Geometry check sheet. Reference: the model listing, model coordinates, mm. Face numbers are marked on the shaded views. A direction names the side the tool comes from. Coordinates: 2 decimals unless noted, no trailing zeros. Write each loop counter-clockwise with the first axis right and the second up, starting at its lowest first coordinate (ties: lowest second). Pieces come first, ordered by that corner, then holes. Notation, with made-up numbers: (84, 27) - (124, 27) arc R13 cw to (124, 51) - close; hole circle Ø2 at (-33.5, 89). An arc over 180 degrees is marked (long way). Answer as a JSON object with one key per item and string values. Group by question number.
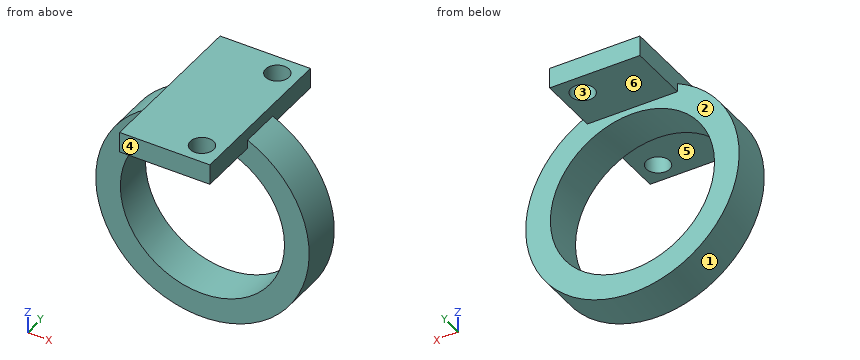
Autodesk Inventor part; units mm, degrees
ref_plane "Work Plane1" through (0, 0, 12) normal (0, 0, 1) x (1, 0, 0)
ref_plane "YZ Plane" through (0, 0, 0) normal (1, 0, 0) x (0, 1, 0)
ref_plane "XZ Plane" through (0, 0, 0) normal (0, 1, 0) x (-1, 0, 0)
sketch "Sketch2" plane through (0, 0, 0) normal (0, 1, 0) x (-1, 0, 0)
  circle A0 centre (0, 0) radius 10
  circle A1 centre (0, 0) radius 13
  dimension "d7" = 20
  dimension "d8" = 26
extrude "Extrusion1" add sketch "Sketch2" along normal blind 5
sketch "Sketch3" plane through (0, 0, 0) normal (0, 0, 1) x (1, 0, 0)
  point P0 (0, 0)
ref_plane "Work Plane1" through (0, 0, 12) normal (0, 0, 1) x (1, 0, 0)
sketch "Sketch4" plane through (0, 0, 12) normal (0, 0, 1) x (1, 0, 0)
  point P0 (0, 0)
sketch "Sketch5" plane through (0, 0, 12) normal (0, 0, 1) x (1, 0, 0)
  line L0 (-13, 0) -> (13, 0)
  line L1 (5.5, 0) -> (-5.5, 0)
  line L2 (-5.5, 0) -> (-5.5, 12.5)
  line L3 (-5.5, 12.5) -> (5.5, 12.5)
  line L4 (5.5, 12.5) -> (5.5, 0)
  line L5 (-5.5, 0) -> (5.5, 0)
  line L6 (5.5, 0) -> (5.5, -7.5)
  line L7 (5.5, -7.5) -> (-5.5, -7.5)
  line L8 (-5.5, -7.5) -> (-5.5, 0)
  line L9 (0, -16.9) -> (0, 20.9)
  dimension "d16" = 11
  dimension "d17" = 7.5
  dimension "d18" = 12.5
  dimension "d19" = 5.5
extrude "Extrusion2" add sketch "Sketch5" along normal mid plane 2.5
sketch "Sketch6" plane through (0, 0, 13.25) normal (0, 0, 1) x (1, 0, 0)
  line L0 (5.5, -7.5) -> (5.5, 12.5)
  line L1 (5.5, 12.5) -> (-5.5, 12.5)
  line L2 (-5.5, -7.5) -> (5.5, -7.5)
  point P0 (0, 0)
  point P1 (3, 10)
  point P2 (3, -5)
  dimension "d20" = 2.5
  dimension "d21" = 2.5
  dimension "d22" = 2.5
  dimension "d30" = 2.5
hole "Hole1" at (3, -5, 13.25) at (3, 10, 13.25) direction (0, 0, -1) diameter 2.85 depth 8 tip angle 118
properties part number "Ring"
(1) Gauge pin test, flat ends, axial feed: pin 1 (1.5 mm diameter, centred on y = 0, z = 7.5, fed in from +X); pin 2 (7.5 mm diameter, centred on x = -2, z = -6.5, fed in from +Y); pin 3 (2 mm diameter, centred on y = 3.5, z = -9, fed in from -X). Record the tip position at first contact, or that the pin passes through.
(2) Draft check along X on the marked faces 1, 2 and 3. Enter one of: +X half, -X half, draft (parallel to the pull), parting line (faces both ways), or undercut.
(3) Section check C-C (z = 0). Record the cut outline in (x, y), and give its area (3 significant figures).
(4) Section check D-D (x = 3). Record the cut outline in (y, z) (3 decimals), and give its area (3 significant figures).
(5) Section check A-A (x = 0). Record the cut outline in (y, z).
(6) Material ranges on L1, parallel to Y at x = 3, z = 12.6 (3 decimals); L2, parallel to X at y = -5, z = 12.5 (3 decimals); L3, parallel to Z at x = 0, y = 1.2, recorded low to high. Write a range as [from, to].
(7) Section check B-B (y = -5). Record the cut outline in (x, z) (3 decimals), and give its area (3 significant figures).
(8) Set-up check for the marked faces 4, 5 and 6: record each of +Z, -Z, +X, -X, +Y, -Y from which the full face is reachable in a straight line by a thin tool's end or side.
Conclusion:
{
 "1": {"pin 1": "stops at x = 11.11", "pin 2": "stops at y = 5", "pin 3": "stops at x = -10.25"},
 "2": {"face 1": "parting line", "face 2": "draft", "face 3": "undercut"},
 "3": {"outline": "(-13, 0) - (-10, 0) - (-10, 5) - (-13, 5) - close; (10, 0) - (13, 0) - (13, 5) - (10, 5) - close", "area": "30.0 mm^2"},
 "4": {"outline": "(-7.5, 10.75) - (-6.425, 10.75) - (-6.425, 13.25) - (-7.5, 13.25) - close; (-3.575, 10.75) - (0, 10.75) - (0, 9.539) - (5, 9.539) - (5, 10.75) - (8.575, 10.75) - (8.575, 13.25) - (-3.575, 13.25) - close; (0, -12.649) - (5, -12.649) - (5, -9.539) - (0, -9.539) - close; (11.425, 10.75) - (12.5, 10.75) - (12.5, 13.25) - (11.425, 13.25) - close", "area": "57.4 mm^2"},
 "5": {"outline": "(-7.5, 10.75) - (0, 10.75) - (0, 10) - (5, 10) - (5, 10.75) - (12.5, 10.75) - (12.5, 13.25) - (-7.5, 13.25) - close; (0, -13) - (5, -13) - (5, -10) - (0, -10) - close"},
 "6": {"L1": "y = [-7.5, -6.425], [-3.575, 8.575], [11.425, 12.5]", "L2": "x = [-5.5, 1.575], [4.425, 5.5]", "L3": "z = [-13, -10], [10, 13.25]"},
 "7": {"outline": "(-5.5, 10.75) - (1.575, 10.75) - (1.575, 13.25) - (-5.5, 13.25) - close; (4.425, 10.75) - (5.5, 10.75) - (5.5, 13.25) - (4.425, 13.25) - close", "area": "20.4 mm^2"},
 "8": {"face 4": "+Z, -Z, +X, -X, -Y", "face 5": "-Z, +X, -X, -Y", "face 6": "-Z, +X, -X, +Y"}
}
